Here's the drawing with two shaded views (mm, measured from the low corner). I have some questions. A direction names the side the tool comes from. Coordinates: 2 decimals unless noted, no trailing zeros. Order: outer loops, then holes, each group sorted by start corner. A loop starts at its lowest first (then second) coordinate and runs counter-clockwise, first axis right, second up. Notation, with made-up numbers: (-29.5, 49) - (-2.5, 49) arc R25 cw to (-2.5, 82) - close; hole circle Ø4 at (23, 76). An arc over 180 degrees is marked (long way). Answer as a JSON object with one key per item and string values. Group by question number.
(1) Please list where these lines run through material, in increasing order: probe 1 along Z at (x, y) = (18.5, 5.5); probe 2 along Y at (x, z) = (31, 5.5).
(2) Which directions (+Z, -Z, +X, -X, +Y, -Y) give clear straight access to the entire face, cutting with the end or side of a thin tool? Please do the marked faces 1, 2 and 3.
(3) Imagine slicing it at D-D, the plane x = 43. Write out the boundary of the cut face in (y, z).
(4) Imagine slicing it at C-C, the plane x = 33. Write out the boundary of the cut face in (y, z).
(5) Will these pins go through, and if not, where does the flat tip stop? P1, Ø6, axis at x = 33, y = 9.5, coming from the +Z side; P2, Ø6, axis at x = 17, y = 1.5, coming from the +Z side; P3, Ø2, axis at x = 35, y = 4, coming from the -Z side; P4, Ø5.5, axis at y = 5.5, z = 5.5, coming from the -X side.
(6) Imagine slicing it at A-A, the plane y = 5.5. Write out the boundary of the cut face in (x, z) (1 decimal).
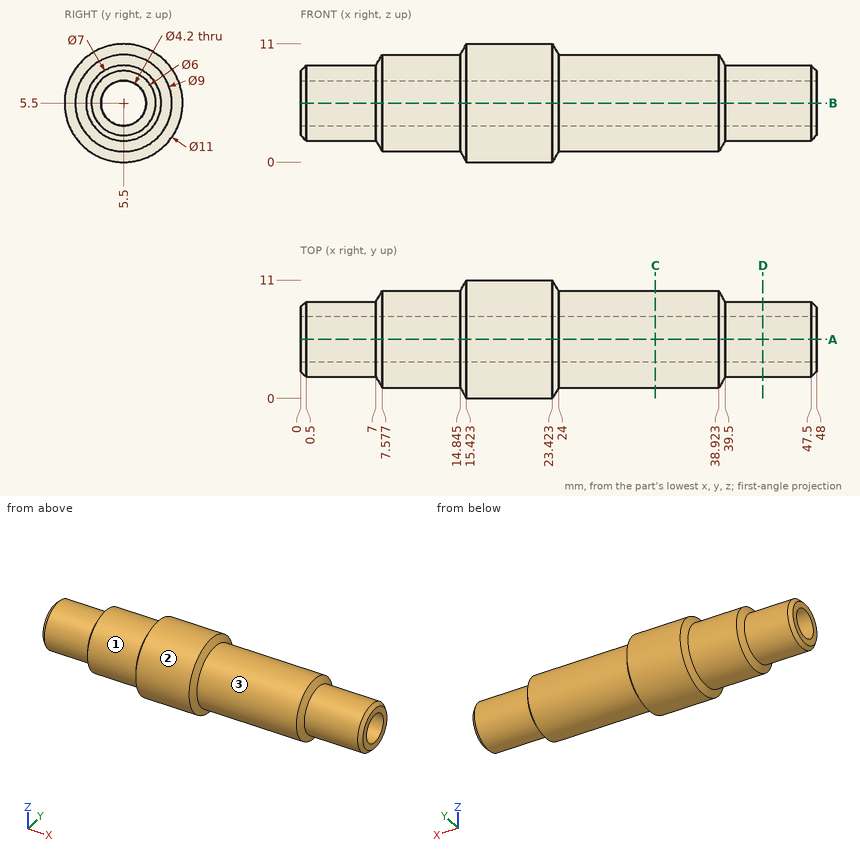
Result set:
{
 "1": {"probe 1": "z = 0 to 3.4, 7.6 to 11", "probe 2": "y = 1 to 3.4, 7.6 to 10"},
 "2": {"face 1": "-X", "face 2": "+X, -X", "face 3": "+X"},
 "3": {"outline": "circle Ø7 at (5.5, 5.5); hole circle Ø4.2 at (5.5, 5.5)"},
 "4": {"outline": "circle Ø9 at (5.5, 5.5); hole circle Ø4.2 at (5.5, 5.5)"},
 "5": {"P1": "stops at z = 9.89", "P2": "stops at z = 10.91", "P3": "stops at z = 1.03", "P4": "stops at x = 0"},
 "6": {"outline": "(0, 2.5) - (0.5, 2) - (7, 2) - (7.6, 1) - (14.8, 1) - (15.4, 0) - (23.4, 0) - (24, 1) - (38.9, 1) - (39.5, 2) - (47.5, 2) - (48, 2.5) - (48, 3.4) - (0, 3.4) - close; (0, 7.6) - (48, 7.6) - (48, 8.5) - (47.5, 9) - (39.5, 9) - (38.9, 10) - (24, 10) - (23.4, 11) - (15.4, 11) - (14.8, 10) - (7.6, 10) - (7, 9) - (0.5, 9) - (0, 8.5) - close"}
}
